```python
from build123d import *

# Parameters (mm, degrees)
SKETCH1_W               = 23
SKETCH1_H               = 15
BOSS_EXTRUDE1_DEPTH     = 35
SKETCH2_W               = 9
SKETCH2_H               = 15
CUT_EXTRUDE1_DEPTH      = 30
CUT_EXTRUDE2_DEPTH      = 45.485952839
CUT_EXTRUDE2_DEPTH_BACK = 45.485952839
SKETCH3_R               = 1.6
CHAMFER1_SIZE           = 2.5
CHAMFER1_SIZE_2         = 14.178204549
SKETCH4_R               = 2.2
CUT_EXTRUDE3_DEPTH      = 10
CUT_EXTRUDE4_DEPTH      = 2
SKETCH6_R               = 3.25
CUT_EXTRUDE5_DEPTH      = 2.5
CUT_EXTRUDE6_DEPTH      = 3.8


with BuildPart() as part:
    # Sketch1 → Boss-Extrude1 (new body)
    with BuildSketch(Plane(origin=(0, 0, 0), x_dir=(0, 0, -1), z_dir=(1, 0, 0))):
        with Locations((11.5, 7.5)):
            Rectangle(SKETCH1_W, SKETCH1_H)
    extrude(amount=BOSS_EXTRUDE1_DEPTH)

    # Sketch2 → Cut-Extrude1 (cut)
    with BuildSketch(Plane(origin=(35, 0, 0), x_dir=(0, 0, -1), z_dir=(1, 0, 0))):
        with Locations((11.5, 7.5)):
            Rectangle(SKETCH2_W, SKETCH2_H)
    extrude(amount=-CUT_EXTRUDE1_DEPTH, mode=Mode.SUBTRACT)

    # Sketch3 → Cut-Extrude2 (cut, two sides: drawn at the far end of the back side and taken through both)
    with BuildSketch(Plane(origin=(0, 0, -23), x_dir=(-1, 0, 0), z_dir=(0, 0, -1)).offset(-CUT_EXTRUDE2_DEPTH_BACK)):
        with Locations(Location((-31, 7.5, 0), (0, 0, 90))):
            Circle(SKETCH3_R)
    extrude(amount=CUT_EXTRUDE2_DEPTH + CUT_EXTRUDE2_DEPTH_BACK, mode=Mode.SUBTRACT)

    # Chamfer1
    # the kernel refuses this chamfer: 14.178204549, 2.5 mm, written as the material it takes off along each edge
    with BuildSketch(Plane(origin=(0, 15, -59.842614584), x_dir=(-0.21013876076743537, -0.9776715712462578, 0), z_dir=(0, 0, 1))) as chamfer1_piece_1:
        Polygon((CHAMFER1_SIZE * 0.977671571246, CHAMFER1_SIZE * 0.210138760767), (-CHAMFER1_SIZE_2 * 0.210138760768, CHAMFER1_SIZE_2 * 0.977671571249), (0, 0), align=None)
    extrude(amount=96.685229169, mode=Mode.SUBTRACT)

    # Sketch4 → Cut-Extrude3 (cut)
    with BuildSketch(Plane.ZY):
        with Locations((-11.5, 6.25)):
            Circle(SKETCH4_R)
    extrude(amount=-CUT_EXTRUDE3_DEPTH, mode=Mode.SUBTRACT)

    # Sketch5 → Cut-Extrude4 (cut)
    with BuildSketch(Plane(origin=(5, 0, 0), x_dir=(0, 0, -1), z_dir=(1, 0, 0))):
        Polygon((7.9, 8.328460969), (7.9, 4.171539031), (11.5, 2.093078062), (15.1, 4.171539031), (15.1, 8.328460969), (11.5, 10.406921938), align=None)
    extrude(amount=-CUT_EXTRUDE4_DEPTH, mode=Mode.SUBTRACT)

    # Sketch6 → Cut-Extrude5 (cut)
    with BuildSketch(Plane(origin=(0, 0, -23), x_dir=(-1, 0, 0), z_dir=(0, 0, -1))):
        with Locations((-31, 7.5)):
            Circle(SKETCH6_R)
    extrude(amount=-CUT_EXTRUDE5_DEPTH, mode=Mode.SUBTRACT)

    # Sketch7 → Cut-Extrude6 (cut)
    with BuildSketch(Plane.XY):
        Polygon((28.15, 9.145448267), (28.15, 5.854551733), (31, 4.209103466), (33.85, 5.854551733), (33.85, 9.145448267), (31, 10.790896534), align=None)
    extrude(amount=-CUT_EXTRUDE6_DEPTH, mode=Mode.SUBTRACT)


solid = part.part
```
Geometry: final body of the model. Coordinates: model frame, mm. A direction names the side the tool comes from. Give positions to 0.01 mm unless a question says otherwise; leave off trailing zeros. Loops run counter-clockwise (first coordinate to the right, second up) from the corner with the lowest first, then second, coordinate; pieces in that order, holes last. Notation, with made-up numbers: (63.5, 74) - (83.5, 74) arc R17 ccw to (83.5, 83) - close; hole circle Ø3 at (39, 43). An arc over 180 degrees is marked (long way). Answer as CSV lines item,"result". Start each with the question number.
(1) Section query D-D (x = 32). Output: boundary loops of the cut face in (y, z).
(2) Section query C-C (z = -4.75). Output: boundary loops of the cut face in (x, y), and give its area (3 significant figures).
(3) Pin query (flat end, axial travel): P1, Ø1, axis at x = 22, z = -14.5, coming from the -Y side; P2, Ø4.5, axis at y = 9, z = -11, coming from the +X side; P3, Ø10, axis at x = 5.5, z = -2.5, coming from the +Y side; P4, Ø4, axis at x = 31, y = 7.5, coming from the +Z side. Return the tip coordinate at first contact, or that it passes through.
(4) Ray query, line 1 along Z through (x, y) = (12, 1.5); line 2 along Y through (x, z) = (31, -21.9); line 3 along X through (y, z) = (7.5, -5). Return the intervals inside material, ascending. Write a range as [from, to].
(5) Section query B-B (y = 1.5). Output: boundary loops of the cut face in (x, z), and give its area (3 significant figures).
(6) Section query A-A (x = 21.5). Output: boundary loops of the cut face in (y, z), and give its area (3 significant figures).
(7) Mould query, pull axis X, two halves, no side actions, for faces 4 (the face through (4, 6, -15.1)), 5 (the face through (29.595, 9.98, -1.873)), 6 (the face through (35, 8, -19)). Classes: +X half, -X half, draft (parallel to the pull), parting line (faces both ways), or undercut.
(8) Reachability of faces 1 (the face through (33.85, 7, -2)), 2 (the face through (20, 7, -7)), 3 (the face through (3, 4, -13)) from +Z, -Z, +X, -X, +Y, -Y: full face, straight path, thin tool, end or side. Return the list, or none.
Worked answers:
1,outline,"(0, -23) - (4.41, -23) - (4.41, -20.5) - (6.25, -20.5) - (6.25, -16) - (0, -16) - close; (0, -7) - (6.25, -7) - (6.25, -3.8) - (4.79, -3.8) - (4.79, 0) - (0, 0) - close; (8.75, -20.5) - (10.59, -20.5) - (10.59, -23) - (15, -23) - (15, -16) - (8.75, -16) - close; (8.75, -7) - (15, -7) - (15, 0) - (10.21, 0) - (10.21, -3.8) - (8.75, -3.8) - close"
2,outline,"(0, 0) - (35, 0) - (35, 15) - (14.18, 15) - (0, 12.5) - close; hole circle Ø3.2 at (31, 7.5)"
2,area,"499 mm^2"
3,P1,"passes through"
3,P2,"stops at x = 5"
3,P3,"stops at y = 14.35"
3,P4,"stops at z = -3.8"
4,line 1,"z = [-23, -16], [-7, 0]"
4,line 2,"y = [0, 4.25], [10.75, 15]"
4,line 3,"x = [0, 29.4], [32.6, 35]"
5,outline,"(0, -23) - (35, -23) - (35, -16) - (5, -16) - (5, -7) - (35, -7) - (35, 0) - (0, 0) - close"
5,area,"535 mm^2"
6,outline,"(0, -23) - (15, -23) - (15, -16) - (0, -16) - close; (0, -7) - (15, -7) - (15, 0) - (0, 0) - close"
6,area,"210 mm^2"
7,face 4,"draft"
7,face 5,"undercut"
7,face 6,"+X half"
8,face 1,"+Z"
8,face 2,"+X, +Y, -Y"
8,face 3,"+X"
